Verification items for the finished model (mm, model axes). Coordinates: 2 decimals unless noted, no trailing zeros. Order: outer loops, then holes, each group sorted by start corner. A loop starts at its lowest first (then second) coordinate and runs counter-clockwise, first axis right, second up. Notation, with made-up numbers: M 18,54.5 L 48,54.5 A23 cw 48,76.5 Z; hole C 9.5,76 d10. An arc over 180 degrees is marked long. Answer as a JSON object with one key per item and string values. Group by question number.
(1) Gauge pin test, flat ends, axial feed: pin 1 Ø5 at (y, z) = (-1, 10) entering from +X; pin 2 Ø4 at (x, z) = (-7.5, 13.5) entering from -Y; pin 3 Ø8 at (x, z) = (-6.5, 5) entering from -Y; pin 4 Ø1 at (x, z) = (1.5, 13) entering from +Y. Record the tip position at first contact, or that the pin passes through.
(2) Cross-section at C-C (y = -14). Enter the section's corners in (x, z), plus the area to 3 significant figures.
(3) Mould release check, pull along Y, two halves, no side actions. Record for faces 1 (the face through (4, -4, 6)), 2 (the face through (-0.54, -2.44, 7.89)), 3 (the face through (-0.867, -3.905, 10.93)): released by +Y, released by -Y, zero draft, split by the parting line, or undercut.
(4) Cross-section at D-D (z = 14.5). Enter the section's corners in (x, y).
(5) Material ranges on line 1 (Y direction, x = 0, z = 4.25); line 2 (Y direction, x = 0, z = 6.5); line 3 (Z direction, x = -12, y = -12.5), recorded low to high.
(6) Cross-section at B-B (x = 3.5). Enter the section's corners in (y, z).
(7) Cross-section at A-A (z = 4.5). Enter the section's corners in (x, y), plus the area to 3 significant figures.
from build123d import *

# Parameters (mm, degrees)
F0_R     = 2.5
F1_DEPTH = 6
F2_R     = 4
F2_R_2   = 2.5
F3_DEPTH = 10


with BuildPart() as f1:
    # F0 (on Top) → F1 (new body)
    with BuildSketch(Plane.XY):
        with BuildLine():
            ThreePointArc((-7.091841, 15.998619), (-9.543133, -14.668967), (17.5, 0))
            ThreePointArc((17.5, 0), (12.271358, 12.476529), (-0.290145, 17.497595))
            ThreePointArc((-0.290145, 17.497595), (-0.27228, 17.294097), (-0.266319, 17.089905))
            ThreePointArc((-0.266319, 17.089905), (-3.213746, 13.633799), (-7.091841, 15.998619))
        make_face()
        Circle(F0_R, mode=Mode.SUBTRACT)
    extrude(amount=F1_DEPTH)

    # F2 (on face) → F3 (join)
    with BuildSketch(Plane.XY.offset(6)):
        Circle(F2_R)
        Circle(F2_R_2, mode=Mode.SUBTRACT)
    extrude(amount=F3_DEPTH)


solid = f1.part
Taken from the geometry:
{
 "1": {"pin 1": "stops at x = 4", "pin 2": "passes through", "pin 3": "stops at y = -17.32", "pin 4": "stops at y = 3.87"},
 "2": {"outline": "M -10.5,0 L 10.5,0 L 10.5,6 L -10.5,6 Z", "area": "126 mm²"},
 "3": {"face 1": "zero draft", "face 2": "undercut", "face 3": "split by the parting line"},
 "4": {"outline": "C 0,0 d8; hole C 0,0 d5"},
 "5": {"line 1": "y = -17.5 to -2.5, 2.5 to 17.5", "line 2": "y = -4 to -2.5, 2.5 to 4", "line 3": "z = 0 to 6"},
 "6": {"outline": "M -17.15,0 L 17.15,0 L 17.15,6 L 1.94,6 L 1.94,16 L -1.94,16 L -1.94,6 L -17.15,6 Z"},
 "7": {"outline": "M -7.09,16 A17.5 ccw long -0.29,17.5 A3.5 cw -0.27,17.09 A3.5 cw Z; hole C 0,0 d5", "area": "924 mm²"}
}
